Drawing for the job (mm, zero at the part's lowest x, y, z). A direction names the side the tool comes from. Coordinates: 2 decimals unless noted, no trailing zeros. Order: outer loops, then holes, each group sorted by start corner. A loop starts at its lowest first (then second) coordinate and runs counter-clockwise, first axis right, second up.
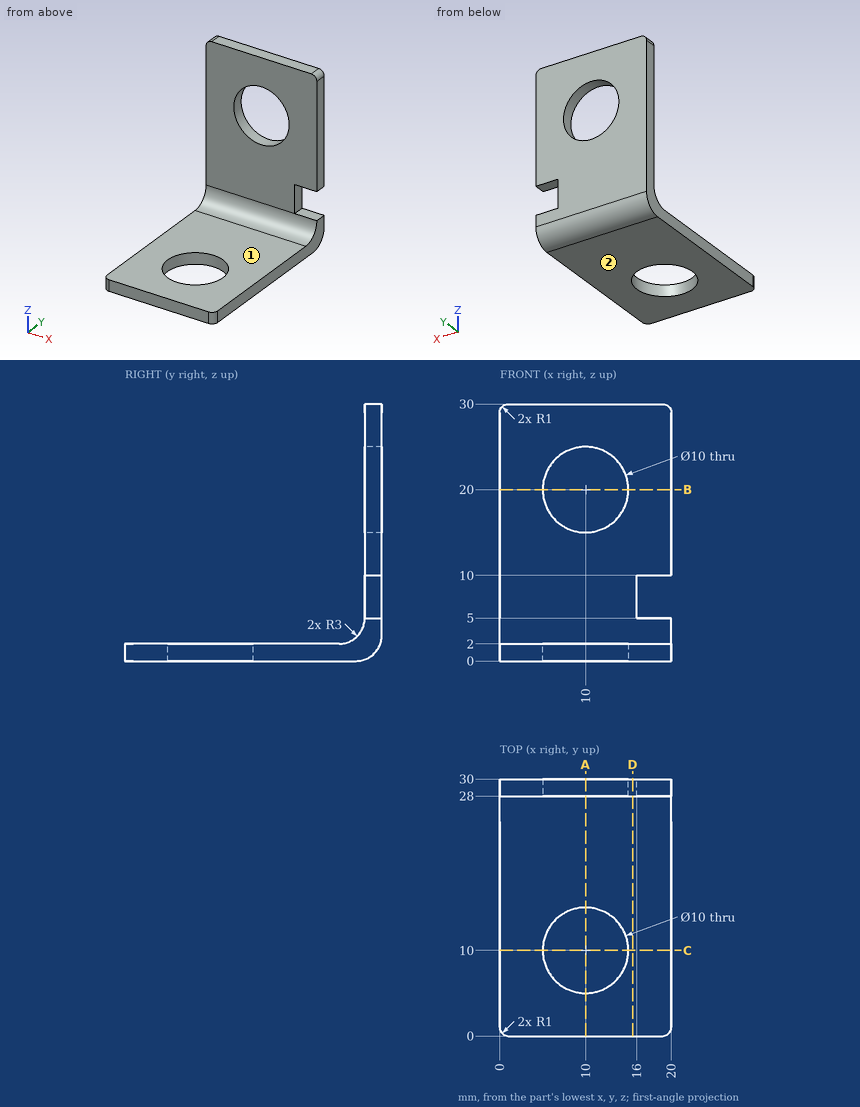
1) Which spindle directions (+Z, -Z, +X, -X, +Y, -Y) get a long thin tool onto all of the face, cutting with end or side? Do the marked faces 1 and 2. Say none if no direction does.
2) Slice it at C-C (y = 10). List the corners of the cut face in (x, z).
3) Slice it at A-A (x = 10). List the corners of the cut face in (y, z).
4) Slice it at D-D (x = 15.5). List the corners of the cut face in (y, z).
5) Drill centre lines: probe 1 along Z at (x, y) = (9.5, 18.25); probe 2 along Y at (x, z) = (7, 28.5); probe 3 along Y at (x, z) = (9.5, 1.25). Where is each one in solid material? Low to high.
6) Slice it at B-B (z = 20). List the corners of the cut face in (x, y).
7) Pin check, flat tips, straight feed: P1, Ø5, axis at x = 8, y = 24.5, coming from the +Z side; P2, Ø1, axis at x = 18, y = 29, coming from the -Z side; P3, Ø1, axis at y = 29, z = 6.5, coming from the +X side. Stop position of each tip, or through.
Worked out:
1. face 1: +Z, +X, -X, -Y
1. face 2: -Z, +X, -X, +Y, -Y
2. outline: (0, 0) - (5, 0) - (5, 2) - (0, 2) - close; (15, 0) - (20, 0) - (20, 2) - (15, 2) - close
3. outline: (0, 0) - (5, 0) - (5, 2) - (0, 2) - close; (15, 0) - (27, 0) arc R3 ccw to (30, 3) - (30, 15) - (28, 15) - (28, 5) arc R3 cw to (25, 2) - (15, 2) - close; (28, 25) - (30, 25) - (30, 30) - (28, 30) - close
4. outline: (0, 0) - (27, 0) arc R3 ccw to (30, 3) - (30, 30) - (28, 30) - (28, 5) arc R3 cw to (25, 2) - (0, 2) - close
5. probe 1: z = 0 to 2
5. probe 2: y = 28 to 30
5. probe 3: y = 0 to 5.03, 14.97 to 29.44
6. outline: (0, 28) - (5, 28) - (5, 30) - (0, 30) - close; (15, 28) - (20, 28) - (20, 30) - (15, 30) - close
7. P1: stops at z = 2.76
7. P2: stops at z = 0.4
7. P3: stops at x = 16
